Input: part model. Units: mm. Frame: model coordinates. A direction names the side the tool comes from. Round coordinates to 2 decimals unless told otherwise and drop trailing zeros. Loops run counter-clockwise (first coordinate to the right, second up) from the corner with the lowest first, then second, coordinate; pieces in that order, holes last. Notation, with made-up numbers: (2, 3.5) - (33, 3.5) arc R21 cw to (33, 30.5) - close; hole circle Ø7 at (-27, 59.25). An arc over 180 degrees is marked (long way). Write each question's results on one line, items separated by ' | '.
from build123d import *

# Parameters (mm, degrees)
SKETCH1_W           = 27.94
SKETCH1_H           = 12.7
BOSS_EXTRUDE1_DEPTH = 6.35
SKETCH2_R           = 4.445
BOSS_EXTRUDE2_DEPTH = 5.842
BOSS_EXTRUDE3_DEPTH = 30.48
SKETCH4_R           = 2.54
BOSS_EXTRUDE4_DEPTH = 7.62
SKETCH5_R           = 2.54
BOSS_EXTRUDE5_DEPTH = 7.62
FILLET1_R           = 2.54


with BuildPart() as part:
    # Sketch1 → Boss-Extrude1 (new body)
    with BuildSketch(Plane(origin=(0, 0, 0), x_dir=(1, 0, 0), z_dir=(0, 1, 0))):
        Rectangle(SKETCH1_W, SKETCH1_H)
    extrude(amount=BOSS_EXTRUDE1_DEPTH)

    # Sketch2 → Boss-Extrude2 (add)
    with BuildSketch(Plane.XZ):
        Circle(SKETCH2_R)
    extrude(amount=BOSS_EXTRUDE2_DEPTH)

    # Sketch3 → Boss-Extrude3 (add)
    with BuildSketch(Plane.XZ):
        with BuildLine():
            Line((-13.97, -6.35), (-13.97, 6.35))
            Line((-13.97, 6.35), (-6.841811913, 6.35))
            ThreePointArc((-6.841811913, 6.35), (-9.3345, 0), (-6.841811913, -6.35))
            Line((-6.841811913, -6.35), (-13.97, -6.35))
        make_face()
        with BuildLine():
            Line((6.841811913, -6.35), (13.97, -6.35))
            Line((13.97, -6.35), (13.97, 6.35))
            Line((13.97, 6.35), (6.841811913, 6.35))
            ThreePointArc((6.841811913, 6.35), (9.3345, 0), (6.841811913, -6.35))
        make_face()
    extrude(amount=BOSS_EXTRUDE3_DEPTH)

    # Sketch4 → Boss-Extrude4 (add)
    with BuildSketch(Plane.ZY.offset(13.97)):
        with Locations((0, -27.94)):
            Circle(SKETCH4_R)
    extrude(amount=BOSS_EXTRUDE4_DEPTH)

    # Sketch5 → Boss-Extrude5 (add)
    with BuildSketch(Plane(origin=(13.97, 0, 0), x_dir=(0, 0, -1), z_dir=(1, 0, 0))):
        with Locations((0, -27.94)):
            Circle(SKETCH5_R)
    extrude(amount=BOSS_EXTRUDE5_DEPTH)

    # Fillet1
    fillet1_edges = [part.edges().sort_by_distance(p)[0] for p in [
        (-13.97, -12.065, -6.35),
        (13.97, -12.065, -6.35),
        (13.97, -12.065, 6.35),
        (-13.97, -12.065, 6.35),
    ]]
    fillet(fillet1_edges, radius=FILLET1_R)


solid = part.part
1. Section query B-B, the plane y = -9.5. Output: boundary loops of the cut face in (x, z).
Answer:
outline: (-13.97, -3.81) arc R2.54 ccw to (-11.43, -6.35) - (-6.84, -6.35) arc R9.33 cw to (-6.84, 6.35) - (-11.43, 6.35) arc R2.54 ccw to (-13.97, 3.81) - close; (6.84, -6.35) - (11.43, -6.35) arc R2.54 ccw to (13.97, -3.81) - (13.97, 3.81) arc R2.54 ccw to (11.43, 6.35) - (6.84, 6.35) arc R9.33 cw to start
2. Mould query, pull axis X, two halves, no side actions, for faces 4 (the flat face through (8, -8, -6.35)), 5 (the flat face through (1.9, 0, -4.3)), 6 (the cylindrical face through (-13.206, -12.323, -5.626)). Classes: pulls with the +X half, pulls with the -X half, needs draft (parallel to the pull), parting line crosses it, or undercut.
Answer:
face 4: needs draft | face 5: undercut | face 6: pulls with the -X half
3. Set-up query: faces 1 (the cylindrical face through (-17.73, -25.42, -0.33)), 2 (the cylindrical face through (9.334, -15.027, 0.098)), 3 (the cylindrical face through (17.73, -25.42, 0.33)). Return all of +Z, -Z, +X, -X, +Y, -Y with unobstructed straight access to the full face (end or side cutting, diameter ignored); none if empty.
Answer:
face 1: -X | face 2: -Y | face 3: +X
4. Contact query for flat-ended pins moving along their axis: pin 1 (6 mm diameter, centred on y = -16, z = 1.5, fed in from +X); pin 2 (6.5 mm diameter, centred on x = 1.5, z = 0, fed in from -Y); pin 3 (6 mm diameter, centred on y = -14.5, z = -0.5, fed in from -X). Output: stop coordinate, or through.
Answer:
pin 1: x = 13.97 | pin 2: y = -5.84 | pin 3: x = -13.97
5. Section query A-A, the plane y = -3. Count the separate pieces of the cut face and the enclosed holes in it, plus the area to 3 significant figures.
Answer:
separate pieces: 3 | enclosed holes: 0 | area: 194 mm^2
6. Section query C-C, the plane x = 0. Output: boundary loops of the cut face in (y, z) (3 decimals), plus the area to 3 significant figures.
Answer:
outline: (-5.842, -4.445) - (0, -4.445) - (0, -6.35) - (6.35, -6.35) - (6.35, 6.35) - (0, 6.35) - (0, 4.445) - (-5.842, 4.445) - close | area: 133 mm^2
7. Section query D-D, the plane y = -27.94. Output: boundary loops of the cut face in (x, z).
Answer:
outline: (-21.59, -2.54) - (-13.97, -2.54) - (-13.97, -3.81) arc R2.54 ccw to (-11.43, -6.35) - (-6.84, -6.35) arc R9.33 cw to (-6.84, 6.35) - (-11.43, 6.35) arc R2.54 ccw to (-13.97, 3.81) - (-13.97, 2.54) - (-21.59, 2.54) - close; (6.84, -6.35) - (11.43, -6.35) arc R2.54 ccw to (13.97, -3.81) - (13.97, -2.54) - (21.59, -2.54) - (21.59, 2.54) - (13.97, 2.54) - (13.97, 3.81) arc R2.54 ccw to (11.43, 6.35) - (6.84, 6.35) arc R9.33 cw to start
8. Line query: line 1 (X direction, y = -7, z = 0); line 2 (X direction, y = -4, z = -3.5); line 3 (X direction, y = -5.5, z = -0.75). Output: solid intervals per line, ascending. Write a range as [from, to].
Answer:
line 1: [-13.97, -9.33], [9.33, 13.97] | line 2: [-13.97, -8.65], [-2.74, 2.74], [8.65, 13.97] | line 3: [-13.97, -9.3], [-4.38, 4.38], [9.3, 13.97]
